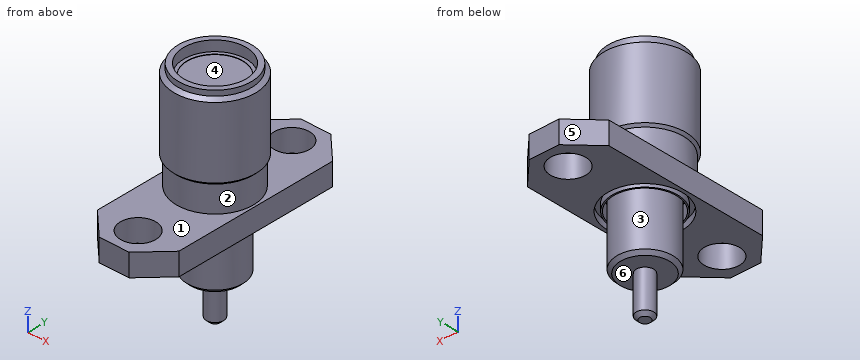
```python
from build123d import *

# Parameters (mm, degrees)
SKETCH_R          = 1.3
SKETCH_R_2        = 2.3
PAD_DEPTH         = 1.65
SKETCH002_R       = 2.75
SKETCH002_R_2     = 2.4
POCKET_DEPTH      = 0.5
SKETCH003_R       = 2.05
SKETCH003_R_2     = 0.635
PAD001_DEPTH      = 8.75
PAD001_DEPTH_BACK = 4
SKETCH004_R       = 0.635
PAD002_DEPTH      = 8.75
PAD002_DEPTH_BACK = 7
CHAMFER_SIZE      = 0.25


with BuildPart() as part:
    # Sketch → Pad (new body)
    with BuildSketch(Plane.XY):
        Polygon((-3, 6.1), (-3, -6.1), (-1.1, -8), (1.1, -8), (3, -6.1), (3, 6.1), (1.1, 8), (-1.1, 8), align=None)
        with Locations((0, 6.1)):
            Circle(SKETCH_R, mode=Mode.SUBTRACT)
        with Locations((0, -6.1)):
            Circle(SKETCH_R, mode=Mode.SUBTRACT)
        Circle(SKETCH_R_2, mode=Mode.SUBTRACT)
    extrude(amount=PAD_DEPTH)

    # Sketch002 → Pocket (cut)
    with BuildSketch(Plane.XY):
        Circle(SKETCH002_R)
        Circle(SKETCH002_R_2, mode=Mode.SUBTRACT)
    extrude(amount=POCKET_DEPTH, mode=Mode.SUBTRACT)

    # Sketch001 → Revolution (revolve)
    with BuildSketch(Plane.YZ):
        Polygon((2.829161, 1.1), (2.829161, 3.579748), (3.003812, 3.754399), (3.003812, 8.938169), (2.6924, 9.14224), (2.6924, 9.53), (2.2987, 9.53), (2.2987, 8.777293), (2.05, 8.777293), (2.05, 1.1), align=None)
    revolve(axis=Axis((0, 0, 0), (0, 0, 1)))

    # Sketch003 → Pad001 (join, two sides)
    with BuildSketch(Plane.XY) as pad001_sk:
        Circle(SKETCH003_R)
        Circle(SKETCH003_R_2, mode=Mode.SUBTRACT)
    extrude(amount=PAD001_DEPTH)
    extrude(pad001_sk.sketch, amount=-PAD001_DEPTH_BACK)

    # Sketch004 → Pad002 (join, two sides)
    with BuildSketch(Plane.XY) as pad002_sk:
        Circle(SKETCH004_R)
    extrude(amount=PAD002_DEPTH)
    extrude(pad002_sk.sketch, amount=-PAD002_DEPTH_BACK)

    # Chamfer
    chamfer_edges = [part.edges().sort_by_distance(p)[0] for p in [
        (-2.05, 0, -4),
        (-0.635, 0, -7),
    ]]
    chamfer(chamfer_edges, length=CHAMFER_SIZE)


solid = part.part
```
Verification items for the finished model (mm, model axes). Face numbers are marked on the shaded views. A direction names the side the tool comes from. Coordinates: 2 decimals unless noted, no trailing zeros. Loops run counter-clockwise (first coordinate to the right, second up) from the corner with the lowest first, then second, coordinate; pieces in that order, holes last. Notation, with made-up numbers: (17, 61) - (65, 61) arc R17 ccw to (65, 78) - close; hole circle Ø8 at (33.25, 6). An arc over 180 degrees is marked (long way). Answer as a JSON object with one key per item and string values.
(1) Scan lines: line 1 along Y through (x, z) = (0, 0.6); line 2 along Z through (x, y) = (-1, 4); line 3 along Z through (x, y) = (1, 0.25). Record each from-to range of solid material in increasing order.
Response:
{"line 1": "y = -8 to -7.4, -4.8 to -2.3, -2.05 to 2.05, 2.3 to 4.8, 7.4 to 8", "line 2": "z = 0 to 1.65", "line 3": "z = -4 to 8.75"}
(2) Cross-section at C-C, the plane x = 0. Count the separate pieces of the cut face and the enclosed holes in it, then the cut area to 3 significant figures.
Response:
{"separate pieces": "3", "enclosed holes": "0", "area": "79.8 mm²"}
(3) Go/stop test with flat-tipped pins: pin 1 Ø1.8 at (y, z) = (2, 1) entering from +X; pin 2 Ø1 at (x, z) = (2.5, 2) entering from -Y; pin 3 Ø0.5 at (y, z) = (3, 0.5) entering from -X. Record where each tip stops, or that it passes through.
Response:
{"pin 1": "stops at x = 3", "pin 2": "stops at y = -6.96", "pin 3": "stops at x = -3"}
(4) Cross-section at A-A, the plane y = -6.5. Record the boundary of the cut face in (x, z), then the cut area to 3 significant figures.
Response:
{"outline": "(-2.6, 0) - (-1.24, 0) - (-1.24, 1.65) - (-2.6, 1.65) - close; (1.24, 0) - (2.6, 0) - (2.6, 1.65) - (1.24, 1.65) - close", "area": "4.50 mm²"}
(5) Access from +Z, -Z, +X, -X, +Y, -Y to the whole of each face (thin tool, end or side, straight path). Record for the marked faces 4, 5 and 6.
Response:
{"face 4": "+Z", "face 5": "+Z, -Z, -X, +Y", "face 6": "-Z"}
(6) Cross-section at B-B, the plane z = -2.5. Record the boundary of the cut face in (x, y), then the cut area to 3 significant figures.
Response:
{"outline": "circle Ø4.1 at (0, 0)", "area": "13.2 mm²"}
(7) Mould release check, pull along Y, two halves, no side actions. Record for the marked faces 1, 2 and 3: pulls with the +Y half, pulls with the -Y half, needs draft (parallel to the pull), parting line crosses it, or undercut.
Response:
{"face 1": "needs draft", "face 2": "parting line crosses it", "face 3": "undercut"}
(8) Cross-section at D-D, the plane y = 7. Record the boundary of the cut face in (x, z).
Response:
{"outline": "(-2.1, 0) - (-0.94, 0) - (-0.94, 1.65) - (-2.1, 1.65) - close; (0.94, 0) - (2.1, 0) - (2.1, 1.65) - (0.94, 1.65) - close"}
